Check sheet for the drawn part. Datum: minimum x, y, z corner. Units: mm. Coordinates: 2 decimals unless noted, no trailing zeros. Order: outer loops, then holes, each group sorted by start corner. A loop starts at its lowest first (then second) coordinate and runs counter-clockwise, first axis right, second up.
Q1. Depth check by flat-ended pin: P1, Ø1, axis at x = 25, z = 6.5, coming from the -Y side; P2, Ø3, axis at x = 52, y = 25, coming from the +Z side (3 decimals); P3, Ø1, axis at y = 29, z = 3.5, coming from the +X side; P4, Ø2, axis at x = 75.5, z = 1, coming from the +Y side. Enter the tip coordinate at first touch or a pass-through.
Q2. Cross-section at C-C, the plane y = 31.5. Record the boundary of the cut face in (x, z) (3 decimals), and give its area (3 significant figures).
Q3. Cross-section at B-B, the plane y = 36. Record the boundary of the cut face in (x, z).
Q4. Cross-section at A-A, the plane x = 26. Record the boundary of the cut face in (y, z) (3 decimals), and give its area (3 significant figures).
Q5. Thickness scan on line 1 (Z direction, x = 36, y = 38); line 2 (Z direction, x = 83, y = 34) (3 decimals); line 3 (Y direction, x = 63, z = 3.25). Record the ranges inside material, lowest first.
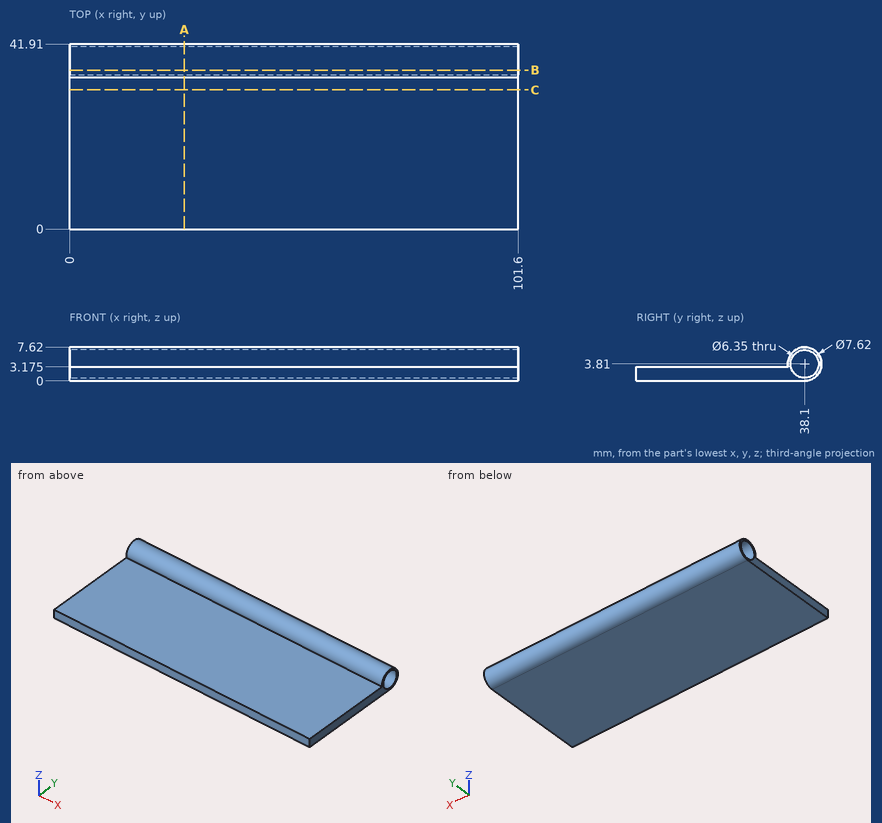
Check values:
1. P1: stops at y = 34.98
1. P2: stops at z = 3.175
1. P3: stops at x = 101.6
1. P4: stops at y = 41.45
2. outline: (0, 0) - (101.6, 0) - (101.6, 3.175) - (0, 3.175) - close
2. area: 323 mm2
3. outline: (0, 0) - (101.6, 0) - (101.6, 1.43) - (0, 1.43) - close; (0, 6.19) - (101.6, 6.19) - (101.6, 6.99) - (0, 6.99) - close
4. outline: (0, 0) - (38.1, 0) arc R3.81 ccw (long way) to (34.343, 3.175) - (0, 3.175) - close; hole circle Ø6.35 at (38.1, 3.81)
4. area: 126 mm2
5. line 1: z = 0 to 0.64, 6.98 to 7.62
5. line 2: z = 0 to 3.175
5. line 3: y = 34.33 to 34.97, 41.23 to 41.87
